The listing builds one solid part. Answer for the finished solid, in the listing's coordinates (mm). A direction names the side the tool comes from. Give positions to 0.01 mm unless a question says otherwise; leave off trailing zeros. Loops run counter-clockwise (first coordinate to the right, second up) from the corner with the lowest first, then second, coordinate; pieces in that order, holes last.
Item 1: A tool of negligible diameter and unlimited length cuts with its end or side. For faces 1 (the face through (0, -2, 3)), 2 (the face through (9.139, 14.334, 0.74)), 3 (the face through (10, 6, 5.5)), from which of +Z, -Z, +X, -X, +Y, -Y can it reach the whole face along a straight path? Write none if from no direction.
Item 2: Consider line 1 along Y through (x, z) = (0, 5.75); line 2 along Y through (x, z) = (0, 1); line 3 along Z through (x, y) = (-10, 7.5). Determine where each line is inside the solid, lowest interval first.
Item 3: The mould has two halves that part along X. Classify faces 4 (the face through (1.617, -0.67, 1.521)), 5 (the face through (-1.5, 11.4, 3.5)), 6 (the face through (4, 0, 0)): pulls with the +X half, pulls with the -X half, needs draft (parallel to the pull), parting line crosses it, or undercut.
Item 4: Each of these flat-tipped pins is pushed along its axis until it touches: pin 1 Ø3 at (y, z) = (6.5, 5) entering from +X; pin 2 Ø4 at (x, z) = (-11.5, 1) entering from +Y. Where does it stop, or does it pass through?
Item 5: Section C-C, the plane z = 6.5 is taken. Give the vertices of the cut face in (x, y).
Item 6: Section D-D, the plane x = -7.5 is taken. Give the vertices of the cut face in (y, z).
Item 7: Section A-A, the plane x = 0 is taken. Give the vertices of the cut face in (y, z).
from build123d import *

# Parameters (mm, degrees)
SKETCH_2_R          = 17
EXTRUDE_1_DEPTH     = 1.5
SKETCH_3_R          = 11.5
EXTRUDE_2_DEPTH     = 4
SKETCH_4_R          = 13.5
EXTRUDE_3_DEPTH     = 1.5
SKETCH_5_R          = 1.75
CUT_EXTRUDE_1_DEPTH = 26.039968051
SKETCH_6_R          = 3
CUT_EXTRUDE_2_DEPTH = 4


with BuildPart() as part:
    # 草图2 → 凸台-拉伸1 (new body)
    with BuildSketch(Plane.XY):
        Circle(SKETCH_2_R)
    extrude(amount=EXTRUDE_1_DEPTH)

    # 草图3 → 凸台-拉伸2 (add)
    with BuildSketch(Plane.XY.offset(1.5)):
        Circle(SKETCH_3_R)
    extrude(amount=EXTRUDE_2_DEPTH)

    # 草图4 → 凸台-拉伸3 (add)
    with BuildSketch(Plane.XY.offset(5.5)):
        Circle(SKETCH_4_R)
    extrude(amount=EXTRUDE_3_DEPTH)

    # 草图5 → 切除-拉伸1 (cut, through all)
    with BuildSketch(Plane.XY.offset(7)):
        Circle(SKETCH_5_R)
    extrude(amount=-CUT_EXTRUDE_1_DEPTH, mode=Mode.SUBTRACT)

    # 草图6 → 切除-拉伸2 (cut)
    with BuildSketch(Plane.XY.offset(7)):
        Circle(SKETCH_6_R)
    extrude(amount=-CUT_EXTRUDE_2_DEPTH, mode=Mode.SUBTRACT)


solid = part.part
Worked answers:
1. face 1: +Z
1. face 2: +Z, -Z
1. face 3: none
2. line 1: y = -13.5 to -3, 3 to 13.5
2. line 2: y = -17 to -1.75, 1.75 to 17
2. line 3: z = 0 to 1.5, 5.5 to 7
3. face 4: undercut
3. face 5: parting line crosses it
3. face 6: needs draft
4. pin 1: stops at x = 12.51
4. pin 2: stops at y = 14.1
5. outline: circle Ø27 at (0, 0); hole circle Ø6 at (0, 0)
6. outline: (-15.26, 0) - (15.26, 0) - (15.26, 1.5) - (8.72, 1.5) - (8.72, 5.5) - (11.22, 5.5) - (11.22, 7) - (-11.22, 7) - (-11.22, 5.5) - (-8.72, 5.5) - (-8.72, 1.5) - (-15.26, 1.5) - close
7. outline: (-17, 0) - (-1.75, 0) - (-1.75, 3) - (-3, 3) - (-3, 7) - (-13.5, 7) - (-13.5, 5.5) - (-11.5, 5.5) - (-11.5, 1.5) - (-17, 1.5) - close; (1.75, 0) - (17, 0) - (17, 1.5) - (11.5, 1.5) - (11.5, 5.5) - (13.5, 5.5) - (13.5, 7) - (3, 7) - (3, 3) - (1.75, 3) - close
